Geometry: final body of the model. Coordinates: model frame, mm. Round coordinates to 2 decimals unless told otherwise and drop trailing zeros. Write each loop counter-clockwise with the first axis right and the second up, starting at its lowest first coordinate (ties: lowest second). Pieces come first, ordered by that corner, then holes.
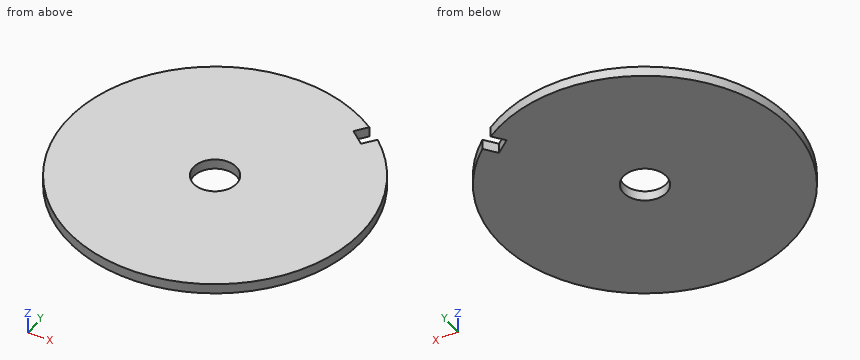
from build123d import *

# Parameters (mm, degrees)
SKETCH1_R               = 92.075
BOSS_EXTRUDE1_DEPTH     = 6.35
CUT_EXTRUDE1_REACH      = 132.368
SKETCH2_R               = 13.49375
CUT_EXTRUDE2_DEPTH      = 131.368453815
CUT_EXTRUDE2_DEPTH_BACK = 131.368453815


with BuildPart() as part:
    # Sketch1 → Boss-Extrude1 (new body)
    with BuildSketch(Plane.XY.offset(3372.777793208)):
        Circle(SKETCH1_R)
    extrude(amount=BOSS_EXTRUDE1_DEPTH)

    # Sketch2 → Cut-Extrude1 (cut, up to next)
    with BuildSketch(Plane.XY.offset(3379.127793208), mode=Mode.PRIVATE) as cut_extrude1_sk1:
        Circle(SKETCH2_R)
    cut_extrude1_tool1 = extrude(cut_extrude1_sk1.sketch, amount=-CUT_EXTRUDE1_REACH, mode=Mode.PRIVATE) & part.part
    add(cut_extrude1_tool1.solids().sort_by_distance((0, 0, 3379.127793))[0], mode=Mode.SUBTRACT)

    # Sketch3 → Cut-Extrude2 (cut, two sides: drawn at the far end of the back side and taken through both)
    with BuildSketch(Plane.XY.offset(3379.127793208).offset(-CUT_EXTRUDE2_DEPTH_BACK)):
        Polygon((337.604296064, 429.104456568), (50.93576887, 76.70301868), (45.174400493, 69.620572204), (54.041166162, 62.407711012), (60.051883822, 69.796682403), (346.720411016, 422.198120291), (895.364622285, 1146.388703686), (886.248507333, 1153.295039963), align=None)
    extrude(amount=CUT_EXTRUDE2_DEPTH + CUT_EXTRUDE2_DEPTH_BACK, mode=Mode.SUBTRACT)


solid = part.part
1) Section D-D on x = 57. Output: boundary loops of the cut face in (y, z) (3 decimals).
2) Line query: probe 1 along Y at (x, z) = (0, 3375.25) (3 decimals); probe 2 along Y at (x, z) = (12, 3377.5); probe 3 along X at (y, z) = (67.5, 3376.5). Output: solid intervals per line, ascending.
3) Section A-A on y = 0. Output: boundary loops of the cut face in (x, z) (3 decimals), plus the area to 3 significant figures.
4) First-contact query: P1, Ø1, axis at y = 59, z = 3376, coming from the -X side; P2, Ø2, axis at x = 26.5, z = 3376, coming from the -Y side; P3, Ø3, axis at y = 57, z = 3374, coming from the +X side. Flat tips, straight axial feed; report the tip coordinate or a pass-through.
Filled in:
1. outline: (-72.31, 3372.778) - (66.045, 3372.778) - (66.045, 3379.128) - (-72.31, 3379.128) - close
2. probe 1: y = -92.075 to -13.494, 13.494 to 92.075
2. probe 2: y = -91.29 to -6.17, 6.17 to 91.29
2. probe 3: x = -62.62 to 47.78, 58.18 to 62.62
3. outline: (-92.075, 3372.778) - (-13.494, 3372.778) - (-13.494, 3379.128) - (-92.075, 3379.128) - close; (13.494, 3372.778) - (92.075, 3372.778) - (92.075, 3379.128) - (13.494, 3379.128) - close
3. area: 998 mm2
4. P1: stops at x = -71.1
4. P2: stops at y = -88.47
4. P3: stops at x = 73.47
